The listing builds one solid part. Answer for the finished solid, in the listing's coordinates (mm). Face numbers are marked on the shaded views. Give positions to 0.01 mm unless a question says otherwise; leave off trailing zeros. Order: outer loops, then holes, each group sorted by start corner. A loop starts at its lowest first (then second) coordinate and runs counter-clockwise, first axis right, second up. Notation, with made-up numbers: (-1, -10.5) - (28, -10.5) arc R27 cw to (28, 25.5) - close; hole circle Ø7 at (71, 69). An arc over 180 degrees is marked (long way). Answer in a Markdown table with one row per item.
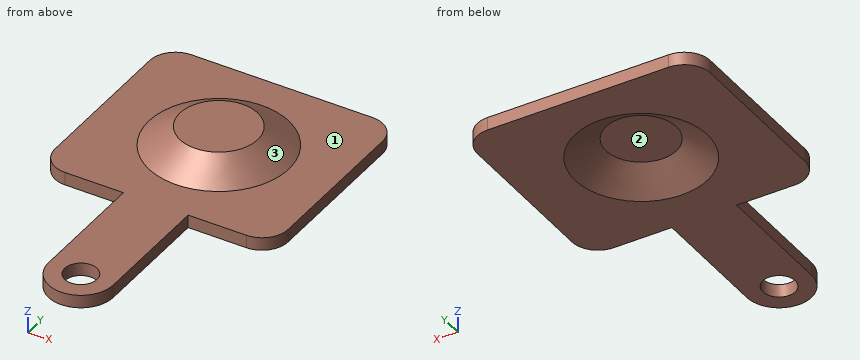
from build123d import *

# Parameters (mm, degrees)
SKETCH1_W           = 9
SKETCH1_H           = 8
BOSS_EXTRUDE1_DEPTH = 0.5
BOSS_EXTRUDE2_DEPTH = 0.5
FILLET1_R           = 1
SKETCH4_R           = 0.625
CUT_EXTRUDE1_DEPTH  = 11.9772492


# Read off the part's stored shape, not the designer's step: Shell1
with BuildPart() as part:
    # Sketch1 → Boss-Extrude1 (new body)
    with BuildSketch(Plane.XY):
        Rectangle(SKETCH1_W, SKETCH1_H)
    extrude(amount=BOSS_EXTRUDE1_DEPTH)

    # Sketch2 → Boss-Extrude2 (add)
    with BuildSketch(Plane.XY):
        with BuildLine():
            Line((1.25, 0), (1.25, -8.75))
            ThreePointArc((1.25, -8.75), (0, -10), (-1.25, -8.75))
            Line((-1.25, -8.75), (-1.25, 0))
            ThreePointArc((-1.25, 0), (0, 1.25), (1.25, 0))
        make_face()
    extrude(amount=BOSS_EXTRUDE2_DEPTH)

    # Fillet1
    fillet1_edges = [part.edges().sort_by_distance(p)[0] for p in [
        (4.5, -4, 0.25),
        (-4.5, -4, 0.25),
        (-4.5, 4, 0.25),
        (4.5, 4, 0.25),
    ]]
    fillet(fillet1_edges, radius=FILLET1_R)

    # Sketch4 → Cut-Extrude1 (cut, through all)
    with BuildSketch(Plane.XY.offset(0.5)):
        with Locations((0, -8.75)):
            Circle(SKETCH4_R)
    extrude(amount=-CUT_EXTRUDE1_DEPTH, mode=Mode.SUBTRACT)

    # Sketch5 → Revolve1 (revolve)
    with BuildSketch(Plane(origin=(0, 0, 0), x_dir=(1, 0, 0), z_dir=(0, 1, 0)), mode=Mode.PRIVATE) as revolve1_sk:
        Polygon((0, -0.5), (2.7, -0.5), (1.5, -1.25), (0, -1.25), align=None)
    revolve(revolve1_sk.sketch.rotate(Axis((0, 0, -88.99), (0, 0, 1)), 180), axis=Axis((0, 0, -88.99), (0, 0, 1)))

    # Shell1 outline → Shell1 (revolve, cut)
    with BuildSketch(Plane.XZ):
        Polygon((2.556601887, 0), (1.356601887, 0.75), (0, 0.75), (0, 0), align=None)
    revolve(axis=Axis((0, 0, 0), (0, 0, 1)), mode=Mode.SUBTRACT)


solid = part.part
Item 1: Determine the mould class of the marked faces 1, 2 and 3 for opening direction Y: pulls with the +Y half, pulls with the -Y half, needs draft (parallel to the pull), parting line crosses it, or undercut.
Answer block:
| item | result |
|---|---|
| face 1 | needs draft |
| face 2 | undercut |
| face 3 | parting line crosses it |
Item 2: Each of these flat-tipped pins is pushed along its axis until it touches: P1, Ø4, axis at x = -3.5, y = 2, coming from the -Z side; P2, Ø3, axis at x = 0.5, y = 0, coming from the -Z side. Where does it stop, or does it pass through?
Answer block:
| item | result |
|---|---|
| P1 | z = 0 |
| P2 | z = 0.35 |
Item 3: Find section C-C on z = 0.3. Write down the section's boundary in (x, y) (3 decimals).
Answer block:
| item | result |
|---|---|
| outline | (-4.5, -3) arc R1 ccw to (-3.5, -4) - (-1.25, -4) - (-1.25, -8.75) arc R1.25 ccw to (1.25, -8.75) - (1.25, -4) - (3.5, -4) arc R1 ccw to (4.5, -3) - (4.5, 3) arc R1 ccw to (3.5, 4) - (-3.5, 4) arc R1 ccw to (-4.5, 3) - close; hole circle Ø4.153 at (0, 0); hole circle Ø1.25 at (0, -8.75) |
Item 4: Find section A-A on x = 0. Write down the section's boundary in (y, z) (3 decimals), then the cut area to 3 significant figures.
Answer block:
| item | result |
|---|---|
| outline | (-10, 0) - (-9.375, 0) - (-9.375, 0.5) - (-10, 0.5) - close; (-8.125, 0) - (-2.557, 0) - (-1.357, 0.75) - (1.357, 0.75) - (2.557, 0) - (4, 0) - (4, 0.5) - (2.7, 0.5) - (1.5, 1.25) - (-1.5, 1.25) - (-2.7, 0.5) - (-8.125, 0.5) - close |
| area | 6.59 mm² |
Item 5: Find section B-B on y = 0. Write down the section's boundary in (x, z).
Answer block:
| item | result |
|---|---|
| outline | (-4.5, 0) - (-2.56, 0) - (-1.36, 0.75) - (1.36, 0.75) - (2.56, 0) - (4.5, 0) - (4.5, 0.5) - (2.7, 0.5) - (1.5, 1.25) - (-1.5, 1.25) - (-2.7, 0.5) - (-4.5, 0.5) - close |
Item 6: Consider line 1 (Y direction, x = 0, z = 0.25) (3 decimals); line 2 (Y direction, x = 0, z = 0.45) (3 decimals); line 3 (Z direction, x = 3.25, y = -3). Determine where each line is inside the solid, lowest interval first.
Answer block:
| item | result |
|---|---|
| line 1 | -10 to -9.375, -8.125 to -2.157, 2.157 to 4 |
| line 2 | -10 to -9.375, -8.125 to -1.837, 1.837 to 4 |
| line 3 | 0 to 0.5 |
